Source: CAD feature listing. Evaluate the final solid. Frame: model axes, mm. Face numbers are marked on the shaded views. A direction names the side the tool comes from. Give positions to 0.01 mm unless a question says otherwise; leave off trailing zeros. Loops run counter-clockwise (first coordinate to the right, second up) from the corner with the lowest first, then second, coordinate; pieces in that order, holes last.
```python
from build123d import *

# Parameters (mm, degrees)
SKETCH2_W           = 88
SKETCH2_H           = 78
BOSS_EXTRUDE1_DEPTH = 20.5
SKETCH5_W           = 84
SKETCH5_H           = 70
CUT_EXTRUDE1_DEPTH  = 18.5
SKETCH6_W           = 4
SKETCH6_H           = 8
CUT_EXTRUDE2_DEPTH  = 18.5
SKETCH7_R           = 1
CUT_EXTRUDE3_DEPTH  = 10
FILLET2_R           = 1


with BuildPart() as part:
    # Sketch2 → Boss-Extrude1 (new body)
    with BuildSketch(Plane.XY):
        Rectangle(SKETCH2_W, SKETCH2_H)
    extrude(amount=BOSS_EXTRUDE1_DEPTH)

    # Sketch5 → Cut-Extrude1 (cut)
    with BuildSketch(Plane.XY.offset(20.5)):
        Rectangle(SKETCH5_W, SKETCH5_H)
    extrude(amount=-CUT_EXTRUDE1_DEPTH, mode=Mode.SUBTRACT)

    # Sketch6 → Cut-Extrude2 (cut)
    with BuildSketch(Plane(origin=(44, 0, 0), x_dir=(0, 0, -1), z_dir=(1, 0, 0))):
        with Locations((-14.4, -12)):
            Rectangle(SKETCH6_W, SKETCH6_H)
    extrude(amount=-CUT_EXTRUDE2_DEPTH, mode=Mode.SUBTRACT)

    # Sketch7 → Cut-Extrude3 (cut)
    with BuildSketch(Plane.XY.offset(20.5)):
        with Locations((-42, 37)):
            Circle(SKETCH7_R)
        with Locations((-42, -37)):
            Circle(SKETCH7_R)
        with Locations((42, -37)):
            Circle(SKETCH7_R)
        with Locations((42, 37)):
            Circle(SKETCH7_R)
    extrude(amount=-CUT_EXTRUDE3_DEPTH, mode=Mode.SUBTRACT)

    # Fillet2
    fillet2_edges = [part.edges().sort_by_distance(p)[0] for p in [
        (44, -39, 10.25),
        (-44, -39, 10.25),
        (-44, 39, 10.25),
        (44, 39, 10.25),
    ]]
    fillet(fillet2_edges, radius=FILLET2_R)


solid = part.part
```
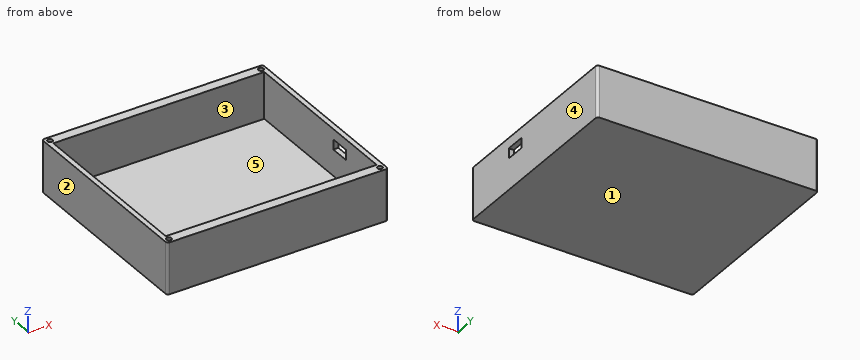
(1) Section A-A, the plane y = -12.5. Return the cut outline in (x, z), then the cut area to 3 significant figures.
A:
outline: (-44, 0) - (44, 0) - (44, 12.4) - (42, 12.4) - (42, 2) - (-42, 2) - (-42, 20.5) - (-44, 20.5) - close; (42, 16.4) - (44, 16.4) - (44, 20.5) - (42, 20.5) - close
area: 242 mm2
(2) Section B-B, the plane z = 6.75. Return the cut outline in (x, y).
A:
outline: (-44, -38) arc R1 ccw to (-43, -39) - (43, -39) arc R1 ccw to (44, -38) - (44, 38) arc R1 ccw to (43, 39) - (-43, 39) arc R1 ccw to (-44, 38) - close; hole (-42, -35) - (42, -35) - (42, 35) - (-42, 35) - close
(3) Mould query, pull axis X, two halves, no side actions, for the marked faces 1, 2 and 3. Classes: pulls with the +X half, pulls with the -X half, needs draft (parallel to the pull), parting line crosses it, or undercut.
A:
face 1: needs draft
face 2: pulls with the -X half
face 3: undercut
(4) Ray query, line 1 along X through (y, z) = (28, 5.5); line 2 along Y through (x, z) = (5.5, 11.25); line 3 along Z through (x, y) = (-18, 0.5). Return the intervals inside material, ascending.
A:
line 1: x = -44 to -42, 42 to 44
line 2: y = -39 to -35, 35 to 39
line 3: z = 0 to 2
(5) First-contact query: pin 1 (1 mm diameter, centred on x = -32.5, y = -21, fed in from +Z); pin 2 (4 mm diameter, centred on x = 31.5, y = -13, fed in from -Z); pin 3 (0.6 mm diameter, centred on x = 42, y = 37, fed in from +Z). Flat tips, straight axial feed; report the tip coordinate or a pass-through.
A:
pin 1: stops at z = 2
pin 2: stops at z = 0
pin 3: stops at z = 10.5
(6) Section D-D, the plane y = 19. Return the cut outline in (x, z), then the cut area to 3 significant figures.
A:
outline: (-44, 0) - (44, 0) - (44, 20.5) - (42, 20.5) - (42, 2) - (-42, 2) - (-42, 20.5) - (-44, 20.5) - close
area: 250 mm2
(7) Reachability of the marked faces 4 and 5 from +Z, -Z, +X, -X, +Y, -Y: full face, straight path, thin tool, end or side. Return the list, or none.
A:
face 4: +Z, -Z, +X, +Y, -Y
face 5: +Z
(8) Section C-C, the plane x = -9.5. Return the cut outline in (y, z).
A:
outline: (-39, 0) - (39, 0) - (39, 20.5) - (35, 20.5) - (35, 2) - (-35, 2) - (-35, 20.5) - (-39, 20.5) - close
